from build123d import *

# Parameters (mm, degrees)
SKETCH_1_W          = 26.5
SKETCH_1_H          = 14.5
EXTRUDE_1_DEPTH     = 3
SKETCH_4_R          = 6
CUT_EXTRUDE_1_DEPTH = 20
SKETCH_5_W          = 36.5
SKETCH_5_H          = 36.5
EXTRUDE_3_DEPTH     = 35
CUT_EXTRUDE_3_DEPTH = 45
SKETCH_9_R          = 2.6
CUT_EXTRUDE_4_DEPTH = 26
FILLET_1_R          = 2
SKETCH_10_R         = 1.6
CUT_EXTRUDE_5_DEPTH = 9
CUT_EXTRUDE_6_DEPTH = 36.5


with BuildPart() as part:
    # 草图1 → 凸台-拉伸1 (new body)
    with BuildSketch(Plane.XY):
        Polygon((29.5, -7), (34.5, -7), (34.5, 35.5), (29.5, 35.5), (-3, 35.5), (-8, 35.5), (-8, -7), (-3, -7), align=None)
        with Locations((13.25, 7.25)):
            Rectangle(SKETCH_1_W, SKETCH_1_H, mode=Mode.SUBTRACT)
    extrude(amount=EXTRUDE_1_DEPTH)

    # 草图4 → 切除-拉伸1 (cut)
    with BuildSketch(Plane.XY.offset(3)):
        with Locations((3.25, 25.5)):
            Circle(SKETCH_4_R)
        with Locations((23.25, 25.5)):
            Circle(SKETCH_4_R)
    extrude(amount=-CUT_EXTRUDE_1_DEPTH, mode=Mode.SUBTRACT)

    # 草图5 → 凸台-拉伸3 (add)
    with BuildSketch(Plane.XY.offset(3)):
        Polygon((-8, 35.5), (-8, 32.5), (-8, -7), (34.5, -7), (34.5, 35.5), align=None)
        with Locations((13.25, 14.25)):
            Rectangle(SKETCH_5_W, SKETCH_5_H, mode=Mode.SUBTRACT)
    extrude(amount=EXTRUDE_3_DEPTH)

    # 草图8 → 切除-拉伸3 (cut)
    with BuildSketch(Plane.ZY.offset(8)):
        Polygon((38, -7), (38, 8), (38, 18), (8, -7), align=None)
    extrude(amount=-CUT_EXTRUDE_3_DEPTH, mode=Mode.SUBTRACT)

    # 草图9 → 切除-拉伸4 (cut)
    with BuildSketch(Plane(origin=(34.5, 0, 0), x_dir=(0, 0, -1), z_dir=(1, 0, 0))):
        with Locations((-17.132149333, 13.627207238)):
            Circle(SKETCH_9_R)
    extrude(amount=-CUT_EXTRUDE_4_DEPTH, mode=Mode.SUBTRACT)

    # 圆角1
    fillet_1_edges = [part.edges().sort_by_distance(p)[0] for p in [
        (-8, 35.5, 19),
        (34.5, 35.5, 19),
        (34.5, -7, 4),
        (-8, -7, 4),
    ]]
    fillet(fillet_1_edges, radius=FILLET_1_R)

    # 草图10 → 切除-拉伸5 (cut)
    with BuildSketch(Plane(origin=(0, 35.5, 0), x_dir=(1, 0, 0), z_dir=(0, 1, 0))):
        with Locations(Location((21.25, -11.5, 0), (0, 0, 270))):
            Circle(SKETCH_10_R)
        with Locations(Location((5.25, -11.5, 0), (0, 0, 270))):
            Circle(SKETCH_10_R)
    extrude(amount=-CUT_EXTRUDE_5_DEPTH, mode=Mode.SUBTRACT)

    # 草图11 → 切除-拉伸6 (cut)
    with BuildSketch(Plane(origin=(-5, 0, 0), x_dir=(0, 0, -1), z_dir=(1, 0, 0))):
        Polygon((-3, -7), (0, -7), (-3, -4), (-14.237966717, -4), (-14.237966717, -7), align=None)
    extrude(amount=CUT_EXTRUDE_6_DEPTH, mode=Mode.SUBTRACT)


solid = part.part
The model under review builds one solid part; all positions refer to its coordinate system, in mm. A direction names the side the tool comes from. Round coordinates to 2 decimals unless told otherwise and drop trailing zeros. Loops run counter-clockwise (first coordinate to the right, second up) from the corner with the lowest first, then second, coordinate; pieces in that order, holes last. Notation, with made-up numbers: (75.5, 0.25) - (119.5, 0.25) arc R24 ccw to (119.5, 11.25) - close; hole circle Ø1 at (-28.75, -10.75). An arc over 180 degrees is marked (long way). Use CSV: the item, a comma, the result in double quotes.
(1) Clearance check with flat-ended pins moving along their axes: P1, Ø15.5, axis at x = 23.25, y = 25.5, coming from the +Z side; P2, Ø1.5, axis at x = 1.5, y = 11, coming from the +Z side; P3, Ø1.5, axis at x = 18, z = 2, coming from the -Y side; P4, Ø11, axis at x = 17, y = 20.5, coming from the +Z side. State where each tip first meets the part, or that it passes through.
Working result:
P1,"stops at z = 38"
P2,"passes through"
P3,"stops at y = -5.75"
P4,"stops at z = 3"
(2) Take a section at A-A, the plane y = 5. Give the boundary of the cut face in (x, z).
Working result:
outline,"(-8, 0) - (0, 0) - (0, 3) - (-5, 3) - (-5, 22.4) - (-8, 22.4) - close; (26.5, 0) - (34.5, 0) - (34.5, 22.4) - (31.5, 22.4) - (31.5, 3) - (26.5, 3) - close"
(3) Machinability: for faces 1 (the cylindrical face through (33.02, 11.09, 17.7)), 2 (the flat face through (13, 14.5, 1)), 3 (the flat face through (31.5, 17, 19)), which of the approach directions +Z, -Z, +X, -X, +Y, -Y give a long, thin tool a straight path to every point of the face, cutting with its end or side? Answer none if there is none.
Working result:
face 1,"+X"
face 2,"+Z, -Z"
face 3,"+Z, -Y"
(4) Take a section at C-C, the plane z = 11.5. Give the boundary of the cut face in (x, y), plus the area to 3 significant figures.
Working result:
outline,"(-8, -4.08) - (-5, -4.08) - (-5, 32.5) - (3.65, 32.5) - (3.65, 35.5) - (-6, 35.5) arc R2 ccw to (-8, 33.5) - close; (6.85, 32.5) - (19.65, 32.5) - (19.65, 35.5) - (6.85, 35.5) - close; (22.85, 32.5) - (31.5, 32.5) - (31.5, -4.08) - (34.5, -4.08) - (34.5, 33.5) arc R2 ccw to (32.5, 35.5) - (22.85, 35.5) - close"
area,"326 mm^2"
(5) Take a section at B-B, the plane y = 25.5. Give the boundary of the cut face in (x, z), plus the area to 4 significant figures.
Working result:
outline,"(-8, 0) - (-2.75, 0) - (-2.75, 3) - (-5, 3) - (-5, 38) - (-8, 38) - close; (9.25, 0) - (17.25, 0) - (17.25, 3) - (9.25, 3) - close; (29.25, 0) - (34.5, 0) - (34.5, 38) - (31.5, 38) - (31.5, 3) - (29.25, 3) - close"
area,"265.5 mm^2"
(6) For line 1 (X direction, y = 9.5, z = 27.5); line 2 (Y direction, x = 3, z = 1); line 3 (X direction, y = 34.5, z = 11.5), list the stretches that pass through material, from the lowest coordinate up.
Working result:
line 1,"x = -8 to -5, 31.5 to 34.5"
line 2,"y = -6 to 0, 14.5 to 19.51, 31.49 to 35.5"
line 3,"x = -7.73 to 3.65, 6.85 to 19.65, 22.85 to 34.23"
(7) Take a section at D-D, the plane x = 5.25. Give the boundary of the cut face in (y, z).
Working result:
outline,"(-7, 0) - (0, 0) - (0, 3) - (-4, 3) - close; (14.5, 0) - (19.84, 0) - (19.84, 3) - (14.5, 3) - close; (31.16, 0) - (35.5, 0) - (35.5, 9.9) - (32.5, 9.9) - (32.5, 3) - (31.16, 3) - close; (32.5, 13.1) - (35.5, 13.1) - (35.5, 38) - (32.5, 38) - close"
(8) The part is to be moulded in two halves that separate along X. For faces 4 (the cylindrical face through (-7.43, 34.9, 18.73)), 5 (the flat face through (34.5, 18, 15)), 6 (the cylindrical face through (22.33, 34.02, 10.32)), say which applies: pulls with the +X half, pulls with the -X half, needs draft (parallel to the pull), parting line crosses it, or undercut.
Working result:
face 4,"pulls with the -X half"
face 5,"pulls with the +X half"
face 6,"undercut"
